Work out the finished part from the listing and answer in its coordinate system (mm). A direction names the side the tool comes from. Coordinates: 2 decimals unless noted, no trailing zeros. Loops run counter-clockwise (first coordinate to the right, second up) from the corner with the lowest first, then second, coordinate; pieces in that order, holes last. Notation, with made-up numbers: (18.5, 78.25) -> (30.5, 78.25) arc R21 ccw to (30.5, 108.25) -> close; hole circle Ø1 at (-25.75, 20). An arc over 180 degrees is marked (long way). Answer as CSV lines item,"result".
```python
from build123d import *

# Parameters (mm, degrees)
SZKIC1_W                    = 45
SZKIC1_H                    = 34
DODANIE_WYCI_GNI_CIE1_DEPTH = 1.8
SZKIC2_R                    = 1.7
WYTNIJ_WYCI_GNI_CIE1_DEPTH  = 1.8
DODANIE_WYCI_GNI_CIE2_DEPTH = 7.5
SZKIC4_W                    = 31
SZKIC4_H                    = 8.6
DODANIE_WYCI_GNI_CIE3_DEPTH = 7.6


with BuildPart() as part:
    # Szkic1 → Dodanie-wyciągnięcie1 (new body)
    with BuildSketch(Plane(origin=(0, 0, 0), x_dir=(1, 0, 0), z_dir=(0, 1, 0))):
        with Locations((-2.969453376, -1.761254019)):
            Rectangle(SZKIC1_W, SZKIC1_H)
    extrude(amount=DODANIE_WYCI_GNI_CIE1_DEPTH)

    # Szkic2 → Wytnij-wyciągnięcie1 (cut)
    with BuildSketch(Plane(origin=(0, 1.8, 0), x_dir=(1, 0, 0), z_dir=(0, 1, 0))):
        with Locations(Location((-22.269453376, -15.561254019, 0), (0, 0, 270))):
            Circle(SZKIC2_R)
        with Locations(Location((16.330546624, -15.561254019, 0), (0, 0, 90))):
            Circle(SZKIC2_R)
        with Locations(Location((16.330546624, 12.038745981, 0), (0, 0, 270))):
            Circle(SZKIC2_R)
        with Locations(Location((-22.269453376, 12.038745981, 0), (0, 0, 90))):
            Circle(SZKIC2_R)
    extrude(amount=-WYTNIJ_WYCI_GNI_CIE1_DEPTH, mode=Mode.SUBTRACT)

    # Szkic3 → Dodanie-wyciągnięcie2 (add)
    with BuildSketch(Plane(origin=(0, 1.8, 0), x_dir=(1, 0, 0), z_dir=(0, 1, 0))):
        Polygon((-18.469453376, -34.093184344), (-18.469453376, -11.961254019), (12.530546624, -12.093184344), (12.530546624, -34.093184344), align=None)
    extrude(amount=DODANIE_WYCI_GNI_CIE2_DEPTH)

    # Szkic4 → Dodanie-wyciągnięcie3 (add)
    with BuildSketch(Plane(origin=(0, 9.3, 0), x_dir=(1, 0, 0), z_dir=(0, 1, 0))):
        with Locations((-2.969453376, -29.793184344)):
            Rectangle(SZKIC4_W, SZKIC4_H)
    extrude(amount=DODANIE_WYCI_GNI_CIE3_DEPTH)


solid = part.part
```
(1) Consider line 1 along Y through (x, z) = (4, 17.5); line 2 along X through (y, z) = (5.5, 13); line 3 along Y through (x, z) = (0.5, 19). Determine where each line is inside the solid, lowest interval first.
Computed values:
line 1,"0 to 9.3"
line 2,"-18.47 to 12.53"
line 3,"1.8 to 9.3"
(2) A cutting plane is placed at B-B, the plane x = -11.5. Write down the section's boundary in (y, z).
Computed values:
outline,"(0, -15.24) -> (1.8, -15.24) -> (1.8, 11.99) -> (9.3, 11.99) -> (9.3, 25.49) -> (16.9, 25.49) -> (16.9, 34.09) -> (1.8, 34.09) -> (1.8, 18.76) -> (0, 18.76) -> close"
(3) A cutting plane is placed at D-D, the plane y = 4.75. Write down the section's boundary in (x, z), and give its area (3 significant figures).
Computed values:
outline,"(-18.47, 11.96) -> (12.53, 12.09) -> (12.53, 34.09) -> (-18.47, 34.09) -> close"
area,"684 mm2"
(4) Flat-ended cylindrical pins translate along their axes: pin 1 Ø3 at (y, z) = (6.5, 26) entering from -X; pin 2 Ø6 at (x, y) = (7.5, 14) entering from -Z; pin 3 Ø5 at (x, z) = (8.5, 19) entering from +Y; pin 4 Ø8 at (x, z) = (-7.5, 6.5) entering from -Y. Find the tip coordinate at first contact, or state that the pin passes through.
Computed values:
pin 1,"x = -18.47"
pin 2,"z = 25.49"
pin 3,"y = 9.3"
pin 4,"y = 0"
(5) A cutting plane is placed at C-C, the plane z = 2.5. Write down the section's boundary in (x, y).
Computed values:
outline,"(-25.47, 0) -> (19.53, 0) -> (19.53, 1.8) -> (-25.47, 1.8) -> close"
(6) A cutting plane is placed at A-A, the plane z = 14.5. Write down the section's boundary in (x, y).
Computed values:
outline,"(-25.47, 0) -> (-23.6, 0) -> (-23.6, 1.8) -> (-25.47, 1.8) -> close; (-20.94, 0) -> (15, 0) -> (15, 1.8) -> (12.53, 1.8) -> (12.53, 9.3) -> (-18.47, 9.3) -> (-18.47, 1.8) -> (-20.94, 1.8) -> close; (17.66, 0) -> (19.53, 0) -> (19.53, 1.8) -> (17.66, 1.8) -> close"
(7) Which of the six approach directions +Z, -Z, +X, -X, +Y, -Y give full straight-line access (tool end or side, diameter ignored) to faces 4 (the face through (-3, 1, 18.761)), 5 (the face through (12.531, 8, 26)), 6 (the face through (-18.469, 8, 26)), 7 (the face through (-3, 13, 25.493)), 8 (the face through (-20.584, 0.913, 15.34))?
Computed values:
face 4,"+Z, +X, -X, -Y"
face 5,"+Z, -Z, +X, +Y"
face 6,"+Z, -Z, -X, +Y"
face 7,"-Z, +X, -X, +Y"
face 8,"+Y, -Y"
(8) For a pull along X with two mould halves and no side action, classify faces 1 (the face through (-3, 1.8, -2)), 2 (the face through (14.8, 0.9, -11.3)), 3 (the face through (19.531, 1, 2)) as pulls with the +X half, pulls with the -X half, needs draft (parallel to the pull), parting line crosses it, or undercut.
Computed values:
face 1,"needs draft"
face 2,"undercut"
face 3,"pulls with the +X half"
